Autodesk Inventor part; units mm, degrees
ref_plane "Work Plane1" through (0, 0, -15) normal (0, 0, 1) x (1, 0, 0)
ref_plane "YZ Plane" through (0, 0, 0) normal (1, 0, 0) x (0, 1, 0)
ref_plane "XZ Plane" through (0, 0, 0) normal (0, 1, 0) x (-1, 0, 0)
sketch "Sketch1" plane through (0, 0, 0) normal (0, 0, 1) x (1, 0, 0)
  line L0 (0, 0) -> (25, 0)
  line L1 (25, 0) -> (25, 40)
  line L2 (25, 40) -> (0, 40)
  line L3 (0, 40) -> (0, 0)
  dimension "d1" = 25
  dimension "d2" = 40
  dimension "d3" = 25
extrude "Extrusion1" add sketch "Sketch1" against normal blind 30
sketch "Sketch2" plane through (25, 0, 0) normal (1, 0, 0) x (0, 0, -1)
  line L0 (0, 0) -> (30, 0)
  circle A0 centre (15, 6.56) radius 2.46
extrude "Extrusion2" cut sketch "Sketch2" against normal blind 30
sketch "Sketch3" plane through (0, 0, 0) normal (-1, 0, 0) x (0, 0, 1)
  line L0 (0, 0) -> (-30, 0)
  line L1 (-25.05, 0) -> (-4.95, 0)
  line L2 (-4.95, 0) -> (-4.95, 33.12)
  line L3 (-4.95, 33.12) -> (-25.05, 33.12)
  line L4 (-25.05, 33.12) -> (-25.05, 0)
  dimension "d11" = 20.1
extrude "Extrusion3" cut sketch "Sketch3" against normal blind 20
sketch "Sketch4" plane through (0, 0, 0) normal (0, -1, 0) x (1, 0, 0)
  line L0 (20, -4.95) -> (20, -25.05)
  line L1 (20, -15) -> (25, -15)
  line L2 (25, 0) -> (25, -30)
  line L3 (20, -8.025) -> (25, -8.025)
  line L4 (25, -8.025) -> (25, -21.975)
  line L5 (25, -21.975) -> (20, -21.975)
  line L6 (20, -21.975) -> (20, -8.025)
  line L7 (20, -8.025) -> (25, -21.975) construction
  line L8 (25, -8.025) -> (20, -21.975) construction
  line L9 (25, -12.54) -> (25, -17.46)
  point P0 (0, 0)
  point P1 (22.5, -15)
  dimension "d14" = 13.95
extrude "Extrusion4" add sketch "Sketch4" along normal blind 15
sketch "Sketch5" plane through (20, 0, 0) normal (-1, 0, 0) x (0, 0, 1)
  circle A0 centre (-15, 6.56) radius 2.46
  circle A1 centre (-15, 6.56) radius 4.7025
  circle A2 centre (-15, 6.56) radius 2.46
  circle A3 centre (-15, 6.56) radius 2.46
  point P0 (0, 0)
  dimension "d17" = 9.405
extrude "Extrusion5" cut sketch "Sketch5" against normal blind 2.1
sketch "Sketch6" plane through (25, 0, 0) normal (1, 0, 0) x (0, 0, -1)
  circle A0 centre (15, 6.56) radius 4.7025
  line L0 (15, 6.56) -> (15, 23.56)
  circle A1 centre (15, 23.56) radius 2.46
  point P0 (0, 0)
  dimension "d20" = 17
  dimension "d21" = 4.92
extrude "Extrusion6" cut sketch "Sketch6" against normal blind 10 contours A1
sketch "Sketch7" plane through (20, 0, 0) normal (-1, 0, 0) x (0, 0, 1)
  circle A0 centre (-15, 23.56) radius 2.46
  circle A1 centre (-15, 23.56) radius 4.7025
  point P0 (0, 0)
  dimension "d24" = 9.405
extrude "Extrusion7" cut sketch "Sketch7" against normal blind 2.1
sketch "Sketch9" plane through (25, 0, 0) normal (1, 0, 0) x (0, 0, -1)
  circle A0 centre (15, 6.56) radius 2.46
  circle A1 centre (15, 6.56) radius 2.46
  circle A2 centre (15, 23.56) radius 2.46
  circle A3 centre (15, 23.56) radius 2.46
  line L0 (30, 40) -> (30, 0)
  line L1 (30, 0) -> (30, 40)
  line L2 (30, 40) -> (0, 40)
  line L3 (0, 40) -> (0, 0)
  line L4 (0, 0) -> (8.025, 0)
  line L5 (21.975, 0) -> (21.975, -15)
  line L6 (21.975, -15) -> (8.025, -15)
  line L7 (8.025, -15) -> (8.025, 0)
  line L8 (0, 0) -> (8.025, 0)
  line L9 (21.975, 0) -> (30, 0)
extrude "Extrusion8" add sketch "Sketch9" along normal blind 5
sketch "Sketch10" plane through (0, 40, 0) normal (0, 1, 0) x (1, 0, 0)
  line L0 (0, 30) -> (30, 30)
  line L1 (30, 0) -> (0, 0)
  line L2 (0, 30) -> (30, 30)
  line L3 (30, 30) -> (30, 0)
  line L4 (30, 0) -> (0, 0)
  line L5 (0, 0) -> (0, 30)
extrude "Extrusion9" add sketch "Sketch10" along normal blind 30
sketch "Sketch12" plane through (30, 0, 0) normal (1, 0, 0) x (0, 0, -1)
  circle A0 centre (15, 6.56) radius 2.46
  line L0 (15, 6.56) -> (15, 15.06)
  circle A1 centre (15, 15.06) radius 2.525
  point P0 (0, 0)
  dimension "d31" = 8.5
  dimension "d33" = 5.05
extrude "Extrusion10" cut sketch "Sketch12" against normal blind 30 contours A1
sketch "Sketch14" plane through (0, 0, 0) normal (0, 0, 1) x (1, 0, 0)
  line L0 (30, 70) -> (0, 70)
  line L1 (0, 70) -> (0, 85)
  line L2 (30, 0) -> (30, 70)
  line L3 (30, 100) -> (30, 70)
  line L4 (-12, 120) -> (15, 120)
  line L5 (-9.5, 118) -> (-7, 110)
  line L6 (-9.5, 118) -> (-12, 120)
  line L7 (-9.5, 102) -> (-7, 110)
  line L8 (-9.5, 102) -> (-12, 100)
  line L9 (30, 105) -> (15, 120)
  line L10 (30, 105) -> (30, 100)
  line L11 (0, 85) -> (0, 100)
  line L12 (0, 100) -> (-12, 100)
  point P0 (0, 0)
  dimension "d60" = 20
  dimension "d64" = 12
extrude "Extrusion12" add sketch "Sketch14" against normal blind 30
sketch "Sketch15" plane through (0, 0, -25.05) normal (-1, 0, 0) x (0, 0, 1)
  line L0 (0, 33.12) -> (20.1, 33.12)
  line L1 (20.1, 33.12) -> (20.1, 0)
  line L2 (0, 33.12) -> (20.1, 33.12)
  line L3 (20.1, 33.12) -> (20.1, 31.1)
  line L4 (20.1, 31.1) -> (0, 31.1)
  line L5 (0, 31.1) -> (0, 33.12)
  point P0 (25.05, 0)
  dimension "d57" = 2.02
extrude "Extrusion13" add sketch "Sketch15" against normal blind 20
sketch "Sketch20" plane through (0, 0, 0) normal (0, 0, 1) x (1, 0, 0)
  line L0 (0, 100) -> (-12, 100)
  line L1 (0, 100) -> (-12, 100)
  line L2 (-12, 100) -> (-9.5, 102)
  line L3 (-12, 100) -> (-9.5, 102)
  line L4 (-9.5, 102) -> (-7, 110)
  line L5 (-9.5, 102) -> (-7, 110)
  line L6 (-7, 110) -> (-9.5, 118)
  line L7 (-7, 110) -> (-9.5, 118)
  line L8 (-9.5, 118) -> (-12, 120)
  line L9 (-9.5, 118) -> (-12, 120)
  line L10 (-12, 120) -> (15, 120)
  line L11 (-12, 120) -> (15, 120)
  line L12 (15, 120) -> (30, 105)
  line L13 (15, 120) -> (30, 105)
  line L14 (30, 105) -> (30, 90)
  line L15 (30, 0) -> (30, 105)
  line L16 (30, 90) -> (0, 90)
  line L17 (0, 90) -> (0, 100)
  point P0 (0, 0)
  dimension "d65" = 15
  dimension "d66" = 30
extrude "Extrusion14" add sketch "Sketch20" along normal blind 45
ref_plane "Work Plane1" through (0, 0, -15) normal (0, 0, 1) x (1, 0, 0)
mirror "Mirror1" about plane through (0, 0, -15) normal (0, 0, 1) of "Extrusion14"
properties part number "rec_b_16mm_x_120mm"
The listing builds one solid part. Answer for the finished solid, in the listing's coordinates (mm). A direction names the side the tool comes from. Coordinates: 2 decimals unless noted, no trailing zeros. Loops run counter-clockwise (first coordinate to the right, second up) from the corner with the lowest first, then second, coordinate; pieces in that order, holes last.
1) Find section C-C on z = 22. Write down the section's boundary in (x, y).
2) Flat-ended cylindrical pins translate along their axes: pin 1 Ø1 at (x, z) = (23.5, 16.5) entering from -Y; pin 2 Ø2 at (x, z) = (20.5, 7.5) entering from +Y; pin 3 Ø12 at (y, z) = (23.56, -15) entering from -X. Find the tip coordinate at first contact, or state that the pin passes through.
3) Determine the mould class of faces 1 (the face through (-8.23, 106.06, -14.16)), 2 (the face through (25.07, 15.171, -12.477)), 3 (the face through (15, 46, -30)), 4 (the face through (9, 105, 45)) for opening direction Z: pulls with the +Z half, pulls with the -Z half, needs draft (parallel to the pull), parting line crosses it, or undercut.
4) Find section D-D on y = 55. Write down the section's boundary in (x, z).
5) Find section B-B on y = 15.06. Write down the section's boundary in (x, z) (3 decimals), then the cut area to 4 significant figures.
6) Find section A-A on z = -15. Give the number of separate pieces and of enclosed holes in the cut face, then the cut area to 3 significant figures.
7) A tool of negligible diameter and unlimited length cuts with its end or side. For faces 5 (the face through (22.1, 21.5, -13)), 6 (the face through (0, 62, -14)), 7 (the face through (20, 8, -20)), 8 (the face through (15, 90, -52)), from which of +Z, -Z, +X, -X, +Y, -Y can it reach the whole face along a straight path? Write none if from no direction.
8) Find the intervals of material crossed by L1, parallel to Z at x = 26, y = 15.06 (3 decimals); L2, parallel to Y at x = 24, z = -15 (3 decimals); L3, parallel to Y at x = 27, z = -15 (3 decimals), in increasing order.
Values:
1. outline: (-12, 100) - (0, 100) - (0, 90) - (30, 90) - (30, 105) - (15, 120) - (-12, 120) - (-9.5, 118) - (-7, 110) - (-9.5, 102) - close
2. pin 1: stops at y = 90
2. pin 2: stops at y = 115.5
2. pin 3: stops at x = 20
3. face 1: needs draft
3. face 2: undercut
3. face 3: pulls with the -Z half
3. face 4: pulls with the +Z half
4. outline: (0, -30) - (30, -30) - (30, 0) - (0, 0) - close
5. outline: (0, -30) - (30, -30) - (30, -17.525) - (20, -17.525) - (20, -25.05) - (0, -25.05) - close; (0, -4.95) - (20, -4.95) - (20, -12.475) - (30, -12.475) - (30, 0) - (0, 0) - close
5. area: 447.5 mm2
6. separate pieces: 4
6. enclosed holes: 0
6. area: 3,020 mm2
7. face 5: -X
7. face 6: +Z, -Z, -X, -Y
7. face 7: -X, -Y
7. face 8: -Z, +X, -X, -Y
8. L1: z = -30 to -17.525, -12.475 to 0
8. L2: y = -15 to 4.1, 9.02 to 12.535, 17.585 to 21.1, 26.02 to 111
8. L3: y = -15 to 4.1, 9.02 to 12.535, 17.585 to 21.1, 26.02 to 108
